```python
from build123d import *

# Parameters (mm, degrees)
F6_R       = 7.5
F3_R       = 10
F0_R       = 9
F7_FACE_R  = 10
F9_DEPTH   = 1.3
F11_R      = 10
F11_R_2    = 9
F12_DEPTH  = 10
F10_R      = 6
F14_DEPTH  = 11.3
F15_R      = 8.5
F14_FACE_R = 6
F13_W      = 2
F13_H      = 2
F17_DEPTH  = 11.3
F18_DEPTH  = 21.3010001


with BuildPart() as f7:
    # F6 (on plane+point) → F7 section 0
    with BuildSketch(Plane.XY.offset(-10)):
        Circle(F6_R)
    # F3 (on plane+point) → F7 section 1
    with BuildSketch(Plane.XY.offset(-3)):
        Circle(F3_R)
    loft()

    # F0 (on Top) → F8 section 0
    with BuildSketch(Plane.XY):
        Circle(F0_R)
    # F7_face (on face) → F8 section 1
    with BuildSketch(Plane.XY.offset(-3)):
        Circle(F7_FACE_R)
    loft()

    # F9 (add): a face of the model
    f9_faces = [f7.faces().sort_by_distance(p)[0] for p in [
        (0, 0, 0),
    ]]
    extrude(f9_faces, amount=F9_DEPTH)

    # F11 (on face) → F12 (join)
    with BuildSketch(Plane.XY.offset(1.3)):
        Circle(F11_R)
        Circle(F11_R_2, mode=Mode.SUBTRACT)
        Circle(F11_R_2)
    extrude(amount=F12_DEPTH)

    # F10 (on face) → F14 (cut, through all)
    with BuildSketch(Plane(origin=(0, 0, -10), x_dir=(1, 0, 0), z_dir=(0, 0, -1))):
        Circle(F10_R)
    extrude(amount=-F14_DEPTH, mode=Mode.SUBTRACT)

    # F15 (on face) → F16 section 0
    with BuildSketch(Plane.XY.offset(11.3)):
        Circle(F15_R)
    # F14_face (on face) → F16 section 1
    with BuildSketch(Plane(origin=(0, 0, 1.3), x_dir=(1, 0, 0), z_dir=(0, 0, -1))):
        Circle(F14_FACE_R)
    loft(mode=Mode.SUBTRACT)

    # F13 (on face) → F17 (cut, through all)
    with BuildSketch(Plane(origin=(0, 0, -10), x_dir=(1, 0, 0), z_dir=(0, 0, -1))):
        with BuildLine():
            Line((-1, 15), (-1, 7.4330343737))
            ThreePointArc((-1, 7.4330343737), (0, 7.5), (1, 7.4330343737))
            Line((1, 7.4330343737), (1, 15))
            Line((1, 15), (-1, 15))
        make_face()
        with BuildLine():
            Line((-1, 7.4330343737), (-1, 1))
            Line((-1, 1), (1, 1))
            Line((1, 1), (1, 2))
            Line((1, 2), (1, 7.4330343737))
            ThreePointArc((1, 7.4330343737), (0, 7.5), (-1, 7.4330343737))
        make_face()
        with BuildLine():
            Line((15, 1), (7.4330343737, 1))
            ThreePointArc((7.4330343737, 1), (7.4832398666, 0.5011198447), (7.5, 0))
            ThreePointArc((7.5, 0), (7.4832398666, -0.5011198447), (7.4330343737, -1))
            Line((7.4330343737, -1), (15, -1))
            Line((15, -1), (15, 1))
        make_face()
        with BuildLine():
            Line((7.4330343737, 1), (1, 1))
            Line((1, 1), (1, -1))
            Line((1, -1), (7.4330343737, -1))
            ThreePointArc((7.4330343737, -1), (7.4832398666, -0.5011198447), (7.5, 0))
            ThreePointArc((7.5, 0), (7.4832398666, 0.5011198447), (7.4330343737, 1))
        make_face()
        with BuildLine():
            Line((-7.4330343737, 1), (-15, 1))
            Line((-15, 1), (-15, -1))
            Line((-15, -1), (-7.4330343737, -1))
            ThreePointArc((-7.4330343737, -1), (-7.5, 0), (-7.4330343737, 1))
        make_face()
        with BuildLine():
            Line((-1, 1), (-7.4330343737, 1))
            ThreePointArc((-7.4330343737, 1), (-7.5, 0), (-7.4330343737, -1))
            Line((-7.4330343737, -1), (-1, -1))
            Line((-1, -1), (-1, 1))
        make_face()
        Rectangle(F13_W, F13_H)
        with BuildLine():
            Line((1, -1), (-1, -1))
            Line((-1, -1), (-1, -7.4330343737))
            ThreePointArc((-1, -7.4330343737), (0, -7.5), (1, -7.4330343737))
            Line((1, -7.4330343737), (1, -2))
            Line((1, -2), (1, -1))
        make_face()
        with BuildLine():
            ThreePointArc((1, -7.4330343737), (0, -7.5), (-1, -7.4330343737))
            Line((-1, -7.4330343737), (-1, -15))
            Line((-1, -15), (1, -15))
            Line((1, -15), (1, -7.4330343737))
        make_face()
    extrude(amount=-F17_DEPTH, mode=Mode.SUBTRACT)

    # F13 (on face) → F18 (cut, through all)
    with BuildSketch(Plane(origin=(0, 0, -10), x_dir=(1, 0, 0), z_dir=(0, 0, -1))):
        with BuildLine():
            Line((7.4330343737, -1), (1, -1))
            Line((1, -1), (1, -2))
            Line((1, -2), (7.2284161474, -2))
            ThreePointArc((7.2284161474, -2), (7.3477569942, -1.5034850031), (7.4330343737, -1))
        make_face()
        with BuildLine():
            Line((7.4330343737, 1), (1, 1))
            Line((1, 1), (1, -1))
            Line((1, -1), (7.4330343737, -1))
            ThreePointArc((7.4330343737, -1), (7.4832398666, -0.5011198447), (7.5, 0))
            ThreePointArc((7.5, 0), (7.4832398666, 0.5011198447), (7.4330343737, 1))
        make_face()
        with BuildLine():
            Line((1, 2), (1, 1))
            Line((1, 1), (7.4330343737, 1))
            ThreePointArc((7.4330343737, 1), (7.3477569942, 1.5034850031), (7.2284161474, 2))
            Line((7.2284161474, 2), (1, 2))
        make_face()
        with BuildLine():
            ThreePointArc((7.2284161474, 2), (7.3477569942, 1.5034850031), (7.4330343737, 1))
            Line((7.4330343737, 1), (15, 1))
            Line((15, 1), (15, 2))
            Line((15, 2), (7.2284161474, 2))
        make_face()
        with BuildLine():
            Line((15, 1), (7.4330343737, 1))
            ThreePointArc((7.4330343737, 1), (7.4832398666, 0.5011198447), (7.5, 0))
            ThreePointArc((7.5, 0), (7.4832398666, -0.5011198447), (7.4330343737, -1))
            Line((7.4330343737, -1), (15, -1))
            Line((15, -1), (15, 1))
        make_face()
        with BuildLine():
            Line((15, -1), (7.4330343737, -1))
            ThreePointArc((7.4330343737, -1), (7.3477569942, -1.5034850031), (7.2284161474, -2))
            Line((7.2284161474, -2), (15, -2))
            Line((15, -2), (15, -1))
        make_face()
    extrude(amount=-F18_DEPTH, mode=Mode.SUBTRACT)


solid = f7.part
```
The listing builds one solid part. Answer for the finished solid, in the listing's coordinates (mm). A direction names the side the tool comes from. Coordinates: 2 decimals unless noted, no trailing zeros. Loops run counter-clockwise (first coordinate to the right, second up) from the corner with the lowest first, then second, coordinate; pieces in that order, holes last. Notation, with made-up numbers: (-7, 75) -> (15, 75) arc R10 ccw to (15, 94) -> close; hole circle Ø8 at (51.5, 11). An arc over 180 degrees is marked (long way). Use one line per item in the form item = value. Start each with the question number.
Item 1: The part is cut by section C-C on y = 0. Determine the outline of the cut face in (x, z).
Item 2: The part is cut by section D-D on z = -1.25. Determine the outline of the cut face in (x, y), then the cut area to 3 significant figures.
Item 3: A tool of negligible diameter and unlimited length cuts with its end or side. For faces 4 (the face through (-4.279, 4.206, -4.429)), 5 (the face through (-8, 1, -4)), 6 (the face through (1, -7, -4)), from which of +Z, -Z, +X, -X, +Y, -Y can it reach the whole face along a straight path? Write none if from no direction.
Item 4: Flat-ended cylindrical pins translate along their axes: pin 1 Ø8 at (x, y) = (-6, -7.5) entering from -Z; pin 2 Ø3 at (y, z) = (7.5, -2.5) entering from -X; pin 3 Ø4.5 at (x, z) = (-7.5, -4) entering from +Y; pin 4 Ø1.2 at (x, z) = (8, 6) entering from +Y. Find the tip coordinate at first contact, or state that the pin passes through.
Item 5: The part is cut by section B-B on z = 1. Determine the outline of the cut face in (x, y), then the cut area to 3 significant figures.
Item 6: Consider L1, parallel to Y at x = 1.75, z = -7; L2, parallel to Y at x = -5.5, z = 8; L3, parallel to X at y = 2.25, z = 4.25. Determine where each line is inside the solid, lowest interval first. Write a range as [from, to].
Item 7: The part is cut by section A-A on x = 0. Determine the outline of the cut face in (y, z).
Item 8: The mould has two halves that part along Z. Classify faces 1 (the face through (4, -5, -10)), 2 (the face through (-1, 7, -4)), 3 (the face through (6.053, 6.66, 0.641)): released by +Z, released by -Z, zero draft, split by the parting line, or undercut.
Answer key:
q1.outline = (-10, 1.3) -> (-6, 1.3) -> (-8.5, 11.3) -> (-10, 11.3) -> close
q2.outline = (-9.36, -1) arc R9.42 ccw to (-1, -9.36) -> (-1, -5.92) arc R6 cw to (-5.92, -1) -> close; (-9.36, 1) -> (-5.92, 1) arc R6 cw to (-1, 5.92) -> (-1, 9.36) arc R9.42 ccw to start; (1, -9.36) arc R9.42 ccw to (9.2, -2) -> (5.66, -2) arc R6 cw to (1, -5.92) -> close; (1, 5.92) arc R6 cw to (5.66, 2) -> (9.2, 2) arc R9.42 ccw to (1, 9.36) -> close
q2.area = 131 mm2
q3.face_4 = +Z, -Z
q3.face_5 = -Z, +X, -X
q3.face_6 = -Z, +Y, -Y
q4.pin_1 = -10
q4.pin_2 = -7.93
q4.pin_3 = 8.36
q4.pin_4 = 6.73
q5.outline = (-8.94, -1) arc R9 ccw to (-1, -8.94) -> (-1, -5.92) arc R6 cw to (-5.92, -1) -> close; (-8.94, 1) -> (-5.92, 1) arc R6 cw to (-1, 5.92) -> (-1, 8.94) arc R9 ccw to start; (1, -8.94) arc R9 ccw to (8.77, -2) -> (5.66, -2) arc R6 cw to (1, -5.92) -> close; (1, 5.92) arc R6 cw to (5.66, 2) -> (8.77, 2) arc R9 ccw to (1, 8.94) -> close
q5.area = 111 mm2
q6.L1 = [-8.39, -5.74], [5.74, 8.39]
q6.L2 = [-8.35, -5.35], [5.35, 8.35]
q6.L3 = [-9.74, -6.35], [6.35, 9.74]
q7.outline = (-10, 1.3) -> (-6, 1.3) -> (-8.5, 11.3) -> (-10, 11.3) -> close; (6, 1.3) -> (10, 1.3) -> (10, 11.3) -> (8.5, 11.3) -> close
q8.face_1 = released by -Z
q8.face_2 = zero draft
q8.face_3 = undercut
